from build123d import *

# Parameters (mm, degrees)
F0_R     = 3.175
F0_W     = 5.842
F0_H     = 12.7
F1_DEPTH = 6.35
F2_DEPTH = 3.048


with BuildPart() as f1:
    # F0 (on Front) → F1 (new body)
    with BuildSketch(Plane.XZ):
        with BuildLine():
            Line((5.842, 0), (0, 0))
            Line((0, 0), (-0.9398, 0))
            ThreePointArc((-0.9398, 0), (-3.195791, -4.549339), (-8.182663, -5.506983))
            Line((-8.182663, -5.506983), (5.842, -9.398))
            Line((5.842, -9.398), (5.842, 0))
        make_face()
        with BuildLine():
            Line((-0.9398, 0), (0, 0))
            Line((0, 0), (0, 12.7))
            Line((0, 12.7), (5.842, 12.7))
            Line((5.842, 12.7), (5.842, 15.24))
            Line((5.842, 15.24), (-0.508, 15.24))
            Line((-0.508, 15.24), (-10.88063, 3.847543))
            ThreePointArc((-10.88063, 3.847543), (-4.591961, 5.329721), (-0.9398, 0))
        make_face()
        with BuildLine():
            ThreePointArc((-8.182663, -5.506983), (-3.195791, -4.549339), (-0.9398, 0))
            ThreePointArc((-0.9398, 0), (-4.591961, 5.329721), (-10.88063, 3.847543))
            ThreePointArc((-10.88063, 3.847543), (-12.145978, -1.583727), (-8.182663, -5.506983))
        make_face()
        with Locations((-6.6548, 0)):
            Circle(F0_R, mode=Mode.SUBTRACT)
        Polygon((5.842, 12.7), (5.842, 0), (66.294, 0), (66.294, 12.7), (56.134, 12.7), (56.134, 10.16), (10.16, 10.16), (10.16, 12.7), align=None)
        with Locations((2.921, 6.35)):
            Rectangle(F0_W, F0_H)
        with Locations((-6.6548, 0)):
            Circle(F0_R)
    extrude(amount=F1_DEPTH)

    # F0 (on Front) → F2 (join)
    with BuildSketch(Plane.XZ):
        with Locations((-6.6548, 0)):
            Circle(F0_R)
        with BuildLine():
            ThreePointArc((-8.182663, -5.506983), (-3.195791, -4.549339), (-0.9398, 0))
            ThreePointArc((-0.9398, 0), (-4.591961, 5.329721), (-10.88063, 3.847543))
            ThreePointArc((-10.88063, 3.847543), (-12.145978, -1.583727), (-8.182663, -5.506983))
        make_face()
        with Locations((-6.6548, 0)):
            Circle(F0_R, mode=Mode.SUBTRACT)
    extrude(amount=F2_DEPTH)


solid = f1.part
CAD build for the part. Positions are in the model's coordinates, mm. A direction names the side the tool comes from. Coordinates: 2 decimals unless noted, no trailing zeros. Loops run counter-clockwise (first coordinate to the right, second up) from the corner with the lowest first, then second, coordinate; pieces in that order, holes last. Notation, with made-up numbers: (7, 25.5) - (34, 25.5) arc R16 cw to (34, 45.5) - close; hole circle Ø9 at (-31.5, -22.5). An arc over 180 degrees is marked (long way). Write item = value, one per line. Start each with the question number.
Q1. Flat gauge pins, fed straight in: pin 1 Ø0.8 at (y, z) = (-4, 11) entering from -X; pin 2 Ø2 at (x, y) = (35, -4.5) entering from +Z; pin 3 Ø2 at (y, z) = (-4.5, 14.5) entering from +X. Where does each tip first touch, or does it go through?
Q2. Drill centre lines: L1, parallel to Z at x = 26, y = -4; L2, parallel to X at y = -4.25, z = 0.25; L3, parallel to X at y = -2.5, z = 3. Where is each one in solid material? Low to high.
Q3. Cut at B-B, the plane x = 36.5. List the corners of the cut face in (y, z), then the cut area to 3 significant figures.
Q4. Cut at A-A, the plane y = -4. List the corners of the cut face in (x, z) (3 decimals).
Q5. Cut at C-C, the plane z = -1.75. List the corners of the cut face in (x, y).
Q6. Pull direction X, two halves, no side cores. Call faces 1 (the flat face through (33, -3, 10.16)), 2 (the flat face through (26, -6.35, 3)), 3 (the flat face through (-5.622, -3.131, 9.624)): pulls with the +X half, pulls with the -X half, needs draft (parallel to the pull), parting line crosses it, or undercut.
Q7. Which spindle directions (+Z, -Z, +X, -X, +Y, -Y) get a long thin tool onto all of the face, cutting with end or side? Do faces 4 (the flat face through (5.842, -3, -5)), 5 (the flat face through (5.842, -3, 14)), 6 (the flat face through (56.134, -3, 11)). Say none if no direction does.
Computed:
q1.pin_1 = -4.73
q1.pin_2 = 10.16
q1.pin_3 = 5.84
q2.L1 = 0 to 10.16
q2.L2 = -12.36 to 66.29
q2.L3 = -11.52 to 66.29
q3.outline = (-6.35, 0) - (0, 0) - (0, 10.16) - (-6.35, 10.16) - close
q3.area = 64.5 mm²
q4.outline = (-10.881, 3.848) arc R5.715 ccw to (-8.183, -5.507) - (5.842, -9.398) - (5.842, 0) - (66.294, 0) - (66.294, 12.7) - (56.134, 12.7) - (56.134, 10.16) - (10.16, 10.16) - (10.16, 12.7) - (5.842, 12.7) - (5.842, 15.24) - (-0.508, 15.24) - close
q5.outline = (-12.1, -6.35) - (5.84, -6.35) - (5.84, 0) - (-12.1, 0) - close
q6.face_1 = undercut
q6.face_2 = needs draft
q6.face_3 = pulls with the -X half
q7.face_4 = -Z, +X, +Y, -Y
q7.face_5 = +Z, +X, +Y, -Y
q7.face_6 = +Z, +Y, -Y
